Geometry check sheet. Reference: the model listing, model coordinates, mm. A direction names the side the tool comes from. Round coordinates to 2 decimals unless told otherwise and drop trailing zeros. Order: outer loops, then holes, each group sorted by start corner. A loop starts at its lowest first (then second) coordinate and runs counter-clockwise, first axis right, second up.
(1) Gauge pin test, flat ends, axial feed: P1, Ø4, axis at x = -20, z = 32, coming from the +Y side; P2, Ø4, axis at x = 19, y = 0, coming from the +Z side; P3, Ø2.5, axis at x = 20, z = 32, coming from the +Y side; P4, Ø17, axis at x = 0, y = 0, coming from the -Z side. Record the tip position at first contact, or that the pin passes through.
(2) Cross-section at B-B on x = -1. Enter the section's corners in (y, z).
(3) Set-up check for faces 1 (the face through (0, 20, 20)), 2 (the face through (-19.031, -12.605, 33.863)), 3 (the face through (-14.56, 15.21, 32.39)): record each of +Z, -Z, +X, -X, +Y, -Y from which the full face is reachable in a straight line by a thin tool's end or side.
(4) Cross-section at D-D on x = -10.5. Enter the section's corners in (y, z).
(5) Draft check along X on faces 4 (the face through (20, 14, 20)), 5 (the face through (22.003, -12.605, 7.369)), 6 (the face through (-5.4, -13.1, 40)). Enter one of: pulls with the +X half, pulls with the -X half, needs draft (parallel to the pull), parting line crosses it, or undercut.
(6) Cross-section at C-C on z = 8. Enter the section's corners in (x, y), and give its area (3 significant figures).
(7) Thickness scan on L1, parallel to Z at x = 20, y = -16.5; L2, parallel to Y at x = 0, z = 30; L3, parallel to Z at x = 21.5, y = -6. Record the ranges inside material, lowest first.
(8) Cross-section at A-A on z = 14. Enter the section's corners in (x, y), and give its area (3 significant figures).
from build123d import *

# Parameters (mm, degrees)
SALIENTE_EXTRUIR2_DEPTH   = 40
CROQUIS4_R                = 14
CORTAR_EXTRUIR2_DEPTH     = 41
TALADRO_ROSCADO_M51_D     = 4.2
TALADRO_ROSCADO_M51_DEPTH = 15
TALADRO_ROSCADO_M51_TIP   = 1.2618073
TALADRO_ROSCADO_M52_D     = 4.2
TALADRO_ROSCADO_M52_DEPTH = 15
TALADRO_ROSCADO_M52_TIP   = 1.2618073
TALADRO_ROSCADO_M53_D     = 4.2
TALADRO_ROSCADO_M53_DEPTH = 15
TALADRO_ROSCADO_M53_TIP   = 1.2618073
CROQUIS20_R               = 2.1
CORTAR_EXTRUIR3_DEPTH     = 15


with BuildPart() as part:
    # Croquis3 → Saliente-Extruir2 (new body)
    with BuildSketch(Plane.XY):
        Polygon((-26, 8), (-14, 20), (14, 20), (26, 8), (26, -20), (-26, -20), align=None)
    extrude(amount=SALIENTE_EXTRUIR2_DEPTH)

    # Croquis4 → Cortar-Extruir2 (cut, through all)
    with BuildSketch(Plane.XY.offset(40)):
        Circle(CROQUIS4_R)
    extrude(amount=-CORTAR_EXTRUIR2_DEPTH, mode=Mode.SUBTRACT)

    # Taladro roscado M51
    with Locations(Plane.XY.offset(40)):
        with Locations((-13.435028843, 13.435028843)):
            Hole(TALADRO_ROSCADO_M51_D / 2, depth=TALADRO_ROSCADO_M51_DEPTH)
            with Locations((0, 0, -(TALADRO_ROSCADO_M51_DEPTH + TALADRO_ROSCADO_M51_TIP / 2))):  # 118° drill point
                Cone(0, TALADRO_ROSCADO_M51_D / 2, TALADRO_ROSCADO_M51_TIP, mode=Mode.SUBTRACT)

    # Taladro roscado M52
    with Locations(Plane.XY.offset(40)):
        with Locations((-19, 0)):
            Hole(TALADRO_ROSCADO_M52_D / 2, depth=TALADRO_ROSCADO_M52_DEPTH)
            with Locations((0, 0, -(TALADRO_ROSCADO_M52_DEPTH + TALADRO_ROSCADO_M52_TIP / 2))):  # 118° drill point
                Cone(0, TALADRO_ROSCADO_M52_D / 2, TALADRO_ROSCADO_M52_TIP, mode=Mode.SUBTRACT)

    # Taladro roscado M53
    with Locations(Plane.XY.offset(40)):
        with Locations((-13.435028843, -13.435028843), (13.435028843, -13.435028843), (19, 0), (13.435028843, 13.435028843)):
            Hole(TALADRO_ROSCADO_M53_D / 2, depth=TALADRO_ROSCADO_M53_DEPTH)
            with Locations((0, 0, -(TALADRO_ROSCADO_M53_DEPTH + TALADRO_ROSCADO_M53_TIP / 2))):  # 118° drill point
                Cone(0, TALADRO_ROSCADO_M53_D / 2, TALADRO_ROSCADO_M53_TIP, mode=Mode.SUBTRACT)

    # Croquis20 → Cortar-Extruir3 (cut)
    with BuildSketch(Plane(origin=(0, -20, 0), x_dir=(1, 0, 0), z_dir=(0, 1, 0))):
        with Locations((-20, -32)):
            Circle(CROQUIS20_R)
        with Locations((20, -32)):
            Circle(CROQUIS20_R)
        with Locations((-20, -8)):
            Circle(CROQUIS20_R)
        with Locations((20, -8)):
            Circle(CROQUIS20_R)
    extrude(amount=CORTAR_EXTRUIR3_DEPTH, mode=Mode.SUBTRACT)


solid = part.part
Found:
1. P1: stops at y = 16
1. P2: stops at z = 24.94
1. P3: stops at y = 15.25
1. P4: passes through
2. outline: (-20, 0) - (-13.96, 0) - (-13.96, 40) - (-20, 40) - close; (13.96, 0) - (20, 0) - (20, 40) - (13.96, 40) - close
3. face 1: +Z, -Z, +X, -X, +Y
3. face 2: -Y
3. face 3: +Z
4. outline: (-20, 0) - (-9.26, 0) - (-9.26, 40) - (-20, 40) - close; (9.26, 0) - (20, 0) - (20, 40) - (9.26, 40) - close
5. face 4: pulls with the +X half
5. face 5: undercut
5. face 6: needs draft
6. outline: (-26, -20) - (-22.1, -20) - (-22.1, -5) - (-17.9, -5) - (-17.9, -20) - (17.9, -20) - (17.9, -5) - (22.1, -5) - (22.1, -20) - (26, -20) - (26, 8) - (14, 20) - (-14, 20) - (-26, 8) - close; hole circle Ø28 at (0, 0)
6. area: 1,190 mm2
7. L1: z = 0 to 5.9, 10.1 to 29.9, 34.1 to 40
7. L2: y = -20 to -14, 14 to 20
7. L3: z = 0 to 6.53, 9.47 to 30.53, 33.47 to 40
8. outline: (-26, -20) - (26, -20) - (26, 8) - (14, 20) - (-14, 20) - (-26, 8) - close; hole circle Ø28 at (0, 0)
8. area: 1,320 mm2
